Autodesk Inventor part; units mm, degrees
ref_plane "YZ Plane" through (0, 0, 0) normal (1, 0, 0) x (0, 1, 0)
ref_plane "XZ Plane" through (0, 0, 0) normal (0, 1, 0) x (-1, 0, 0)
ref_plane "XY Plane" through (0, 0, 0) normal (0, 0, 1) x (1, 0, 0)
sketch "Boceto1" plane through (0, 0, 0) normal (0, 1, 0) x (-1, 0, 0)
  line L0 (0, 0) -> (550, 0)
  line L1 (550, 0) -> (550, -350)
  line L2 (550, -350) -> (0, -350)
  line L3 (0, -350) -> (0, 0)
  line L4 (0, -175) -> (550, -175) construction
  line L5 (275, -350) -> (275, 0) construction
  circle A0 centre (255, -12.5) radius 5
  circle A1 centre (295, -12.5) radius 5
  circle A2 centre (255, -337.5) radius 5
  circle A3 centre (295, -337.5) radius 5
  dimension "d0" = 350
  dimension "d1" = 550
  dimension "d83" = 12.5
  dimension "d84" = 10
  dimension "d85" = 20
  dimension "d88" = 40
  dimension "d95" = 325
extrude "Extrusión10" add sketch "Boceto1" along normal blind 19
sketch "Boceto8" plane through (0, 19, 0) normal (0, 1, 0) x (1, 0, 0)
  line L0 (-550, 0) -> (0, 0) construction
  line L1 (-275, 0) -> (-275, 350) construction
  line L2 (0, 350) -> (-550, 350) construction
  circle A0 centre (-224.5, 200) radius 6.5
  circle A1 centre (-325.5, 200) radius 6.5
  dimension "d102" = 101
  dimension "d103" = 50.5
  dimension "d104" = 13
  dimension "d116" = 150
extrude "Extrusión11" cut sketch "Boceto8" against normal through all
sketch "Boceto9" plane through (0, 0, 0) normal (0, -1, 0) x (1, 0, 0)
  line L0 (0, -305) -> (-550, -305) construction
  line L1 (-550, -350) -> (-550, 0) construction
  line L2 (0, -350) -> (-550, -350) construction
  line L3 (-230, -305) -> (-320, -305) construction
  line L4 (-230, -300) -> (-320, -300)
  line L5 (-320, -310) -> (-230, -310)
  arc A0 (-230, -310) -> (-230, -300) centre (-230, -305) ccw
  arc A1 (-320, -300) -> (-320, -310) centre (-320, -305) ccw
  line L6 (0, 0) -> (0, -350) construction
  line L7 (0, 0) -> (0, -350)
  line L8 (0, -27) -> (-550, -27) construction
  line L9 (-550, 0) -> (0, 0)
  line L10 (-232.5, -27) -> (-317.5, -27) construction
  line L11 (-232.5, -22) -> (-317.5, -22)
  line L12 (-317.5, -32) -> (-232.5, -32)
  arc A2 (-232.5, -32) -> (-232.5, -22) centre (-232.5, -27) ccw
  arc A3 (-317.5, -22) -> (-317.5, -32) centre (-317.5, -27) ccw
  point P0 (-275, -305)
  point P1 (-275, -305)
  point P2 (-275, -27)
  point P3 (-275, -27)
  dimension "d108" = 45
  dimension "d109" = 10
  dimension "d110" = 90
  dimension "d111" = 27
  dimension "d112" = 10
  dimension "d113" = 85
extrude "Extrusión12" cut sketch "Boceto9" against normal through all
sketch "Sketch10" plane through (0, 0, 0) normal (0, -1, 0) x (1, 0, 0)
  line L0 (-135, -169) -> (-125, -169)
  line L1 (-125, -169) -> (-125, -181)
  line L2 (-125, -181) -> (-135, -181)
  line L3 (-135, -181) -> (-135, -169)
  circle A0 centre (-295, -337.5) radius 5
  line L4 (-550, -350) -> (-550, 0)
  circle A1 centre (-255, -337.5) radius 5
  point P0 (0, 0)
  point P1 (-135, -175)
  point P2 (-550, -175)
  dimension "d117" = 10
  dimension "d118" = 12
  dimension "d122" = 120
extrude "Extrusion13" cut sketch "Sketch10" against normal through all contours L0 L1 L2 L3
properties part number "mesa" material "MDF Tablero de fibras de densidad media"
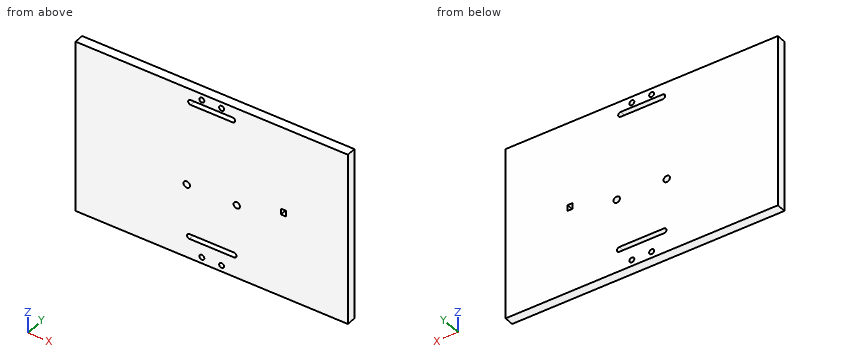
Read the model definition and answer for the solid it produces. Units are mm, in the model's axes. Round coordinates to 2 decimals unless told otherwise and drop trailing zeros. Loops run counter-clockwise (first coordinate to the right, second up) from the corner with the lowest first, then second, coordinate; pieces in that order, holes last.
Q1. Consider probe 1 along Z at (x, y) = (-305, 11.5); probe 2 along X at (y, z) = (5.5, -200); probe 3 along Z at (x, y) = (-255, 13). Determine where each line is inside the solid, lowest interval first.
Q2. This flat-tipped pin is pushed along its axis until it touches: pin 1 (5.5 mm diameter, centred on x = -257.5, y = 12.5, fed in from +Z). Where does it stop, or does it pass through?
Q3. Section A-A on z = -200 is taken. Write down the section's boundary in (x, y).
Output:
1. probe 1: z = -350 to -310, -300 to -32, -22 to 0
1. probe 2: x = -550 to -332, -319 to -231, -218 to 0
1. probe 3: z = -350 to -342.5, -332.5 to -310, -300 to -32, -22 to -17.5, -7.5 to 0
2. pin 1: stops at z = 0
3. outline: (-550, 0) - (-332, 0) - (-332, 19) - (-550, 19) - close; (-319, 0) - (-231, 0) - (-231, 19) - (-319, 19) - close; (-218, 0) - (0, 0) - (0, 19) - (-218, 19) - close
